Autodesk Inventor part; units mm, degrees
ref_plane "YZ Plane" through (0, 0, 0) normal (1, 0, 0) x (0, 1, 0)
ref_plane "XZ Plane" through (0, 0, 0) normal (0, 1, 0) x (-1, 0, 0)
ref_plane "XY Plane" through (0, 0, 0) normal (0, 0, 1) x (1, 0, 0)
sketch "Sketch1" plane through (0, 0, 0) normal (0, 0, 1) x (1, 0, 0)
  line L0 (-20, -37.4) -> (20, -37.4) construction
  line L1 (20, -37.4) -> (20, 37.4) construction
  line L2 (20, 37.4) -> (-20, 37.4) construction
  line L3 (-20, 37.4) -> (-20, -37.4) construction
  line L4 (-20, -37.4) -> (20, 37.4) construction
  line L5 (20, -37.4) -> (-20, 37.4) construction
  line L6 (0, 37.4) -> (0, -37.4) construction
  line L7 (-20, 0) -> (20, 0) construction
  circle A0 centre (0, -17.4) radius 19
  line L8 (8.75, 10.75) -> (-8.75, 10.75)
  line L9 (-8.75, 10.75) -> (-8.75, 28.25)
  line L10 (-8.75, 28.25) -> (8.75, 28.25)
  line L11 (8.75, 28.25) -> (8.75, 10.75)
  line L12 (8.75, 10.75) -> (-8.75, 28.25) construction
  line L13 (-8.75, 10.75) -> (8.75, 28.25) construction
  line L14 (20, 1.6) -> (-20, 1.6) construction
  line L15 (-20, 37.4) -> (-10.85, 37.4) construction
  line L16 (-10.85, 37.4) -> (-10.85, 28.25) construction
  line L17 (-10.85, 28.25) -> (-20, 28.25) construction
  line L18 (-20, 28.25) -> (-20, 37.4) construction
  line L19 (20, 37.4) -> (10.85, 37.4) construction
  line L20 (10.85, 37.4) -> (10.85, 28.25) construction
  line L21 (10.85, 28.25) -> (20, 28.25) construction
  line L22 (20, 28.25) -> (20, 37.4) construction
  line L23 (-10.85, 37.4) -> (-20, 28.25)
  line L24 (-20, -17.4) -> (20, -17.4) construction
  arc A1 (-20, -17.4) -> (20, -17.4) centre (0, -17.4) ccw
  line L25 (-20, 28.25) -> (-20, -17.4)
  line L26 (20, -17.4) -> (20, 28.25)
  line L27 (20, 28.25) -> (10.85, 37.4)
  line L28 (10.85, 37.4) -> (-10.85, 37.4)
  circle A2 centre (0, 19.5) radius 17.9 construction
  circle A3 centre (0, 19.5) radius 10
  line L29 (-8.2219, 35.4) -> (8.2219, 35.4)
  arc A4 (-8.2219, 35.4) -> (8.2219, 35.4) centre (0, 19.5) ccw
  point P0 (0, 0)
  point P1 (0, 1.6)
  point P2 (-10.85, 33.7368)
  point P3 (10.85, 33.7368)
  dimension "d2" = 38
  dimension "d0" = 40
  dimension "d1" = 74.8
  dimension "d3" = 20
  dimension "d4" = 17.5
  dimension "d5" = 17.5
  dimension "d6" = 35.8
  dimension "d7" = 9.15
  dimension "d8" = 9.15
  dimension "d9" = 9.15
  dimension "d10" = 9.15
  dimension "d11" = 9.15
  dimension "d12" = 45.65
  dimension "d21" = 20
  dimension "d22" = 2
extrude "Extrusion1" add sketch "Sketch1" along normal blind 95.7 contours A0
extrude "Extrusion2" add sketch "Sketch1" against normal blind 19 contours L8 A3 L11 | L8 A3 L9 L10 L11 | L8 L9 A3 | A3 L10 L11 | L9 L10 A3
extrude "Extrusion3" add sketch "Sketch1" along normal blind 19 contours A4 L29 | A3 L8 | L11 A3 | A3 L9 | L10 A3 | L28 L27 L26 A1 L25 L23
extrude "Extrusion5" add sketch "Sketch1" along normal blind 182.5 contours A4 L29 | L8 A3 L11 | A3 L8 | L8 A3 L9 L10 L11 | L11 A3 | L8 L9 A3 | A3 L10 L11 | A3 L9 | L10 A3 | L9 L10 A3
extrude "Extrusion6" cut sketch "Sketch1" along normal blind 182.5 contours A3 L8 | L8 A3 L9 L10 L11 | L11 A3 | A3 L9 | L10 A3
extrude "Extrusion7" add sketch "Sketch1" along normal blind 32.5 contours A3 L8 | L8 A3 L9 L10 L11 | L11 A3 | A3 L9 | L10 A3
sketch "Sketch2" plane through (-8.75, 10.75, 0) normal (-1, 0, 0) x (0, 0, 1)
  line L0 (0, 26.65) -> (0, 17.5) construction
  line L1 (0, 0) -> (-19, 0) construction
  line L2 (0, 17.5) -> (-10, 17.5) construction
  line L3 (-10, 17.5) -> (-10, 0) construction
  line L4 (-10, 0) -> (0, 0) construction
  line L5 (0, 0) -> (0, 17.5) construction
  point P0 (0, -10.75)
  point P1 (-10, 8.75)
  dimension "d29" = 10
hole "Hole1" at (-8.75, 19.5, -10) direction (1, 0, 0) diameter 6 end through all both
equation "\"d5\" = d4"
equation "\"d7\" = 0.5 * d6 - 0.5 * d4"
equation "\"d9\" = d8"
equation "\"d10\" = d9"
equation "\"d11\" = d10"
properties part number "actuator_base" material "Aluminum 6061"
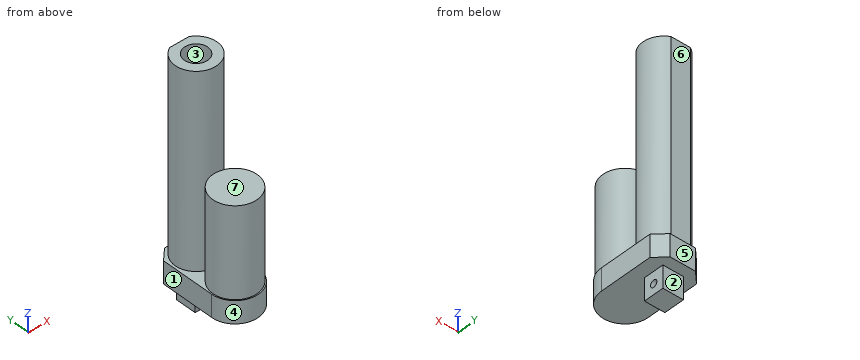
Geometry check sheet. Reference: the model listing, model coordinates, mm. Face numbers are marked on the shaded views. A direction names the side the tool comes from. Coordinates: 2 decimals unless noted, no trailing zeros. Order: outer loops, then holes, each group sorted by start corner. A loop starts at its lowest first (then second) coordinate and runs counter-clockwise, first axis right, second up. Notation, with made-up numbers: (9, -5.5) - (66, -5.5) arc R35 ccw to (66, 31.5) - close; hole circle Ø10 at (-23, 89). An arc over 180 degrees is marked (long way). Answer in a Markdown table with one row per item. Add a question column.
1. Draft check along Y on the marked faces 1, 2, 3 and 4. Enter one of: +Y half, -Y half, draft (parallel to the pull), parting line (faces both ways), or undercut.
2. Section check C-C (z = 34.5). Enter the section's corners in (x, y).
3. Gauge pin test, flat ends, axial feed: pin 1 Ø5 at (x, y) = (5.5, 10.5) entering from -Z; pin 2 Ø6 at (x, y) = (1.5, 19.5) entering from +Z; pin 3 Ø9 at (x, z) = (-4, -7.5) entering from +Y; pin 4 Ø12 at (y, z) = (28, 157.5) entering from -X. Record the tip position at first contact, or that the pin passes through.
4. Section check A-A (y = 19.5). Enter the section's corners in (x, z).
5. Section check D-D (y = 5). Enter the section's corners in (x, z), plus the area to 3 significant figures.
6. Access from +Z, -Z, +X, -X, +Y, -Y to the whole of each face (thin tool, end or side, straight path). Record for the marked faces 5, 6 and 7.
7. Material ranges on L1, parallel to X at y = 19.5, z = 134; L2, parallel to Y at x = 1, z = -10; L3, parallel to Y at x = 0, z = 102, recorded low to high. Write a range as [from, to].
Data:
| question | item | result |
|---|---|---|
| 1 | face 1 | draft |
| 1 | face 2 | +Y half |
| 1 | face 3 | undercut |
| 1 | face 4 | -Y half |
| 2 | outline | circle Ø38 at (0, -17.4); (-8.22, 35.4) arc R17.9 ccw (long way) to (8.22, 35.4) - close; hole circle Ø20 at (0, 19.5) |
| 3 | pin 1 | stops at z = -19 |
| 3 | pin 2 | stops at z = 32.5 |
| 3 | pin 3 | stops at y = 28.25 |
| 3 | pin 4 | stops at x = -17.72 |
| 4 | outline | (-20, 0) - (-8.75, 0) - (-8.75, -7) - (8.75, -7) - (8.75, 0) - (20, 0) - (20, 19) - (17.9, 19) - (17.9, 182.5) - (10, 182.5) - (10, 32.5) - (-10, 32.5) - (-10, 182.5) - (-17.9, 182.5) - (-17.9, 19) - (-20, 19) - close; (-8.75, -19) - (8.75, -19) - (8.75, -13) - (-8.75, -13) - close |
| 5 | outline | (-20, 0) - (20, 0) - (20, 19) - (10.5, 19) - (10.5, 182.5) - (-10.5, 182.5) - (-10.5, 19) - (-20, 19) - close |
| 5 | area | 4,190 mm² |
| 6 | face 5 | +Z, -Z, +X, -X, +Y |
| 6 | face 6 | +Z, +X, -X, +Y |
| 6 | face 7 | +Z, +X, -X, -Y |
| 7 | L1 | x = [-17.9, -10], [10, 17.9] |
| 7 | L2 | y = [10.75, 16.5], [22.5, 28.25] |
| 7 | L3 | y = [1.6, 9.5], [29.5, 35.4] |
